Work out the finished part from the listing and answer in its coordinate system (mm). A direction names the side the tool comes from. Give positions to 0.01 mm unless a question says otherwise; leave off trailing zeros. Write each loop counter-clockwise with the first axis right and the second up, starting at its lowest first coordinate (ties: lowest second). Pieces come first, ordered by that corner, then holes. Notation, with made-up numbers: (19.5, -11.5) - (33.5, -11.5) arc R16 cw to (33.5, -3.5) - close; hole circle Ø8 at (41.25, 84). An arc over 180 degrees is marked (long way). Write each question's results on one line, items separated by ' | '. Start each with the question number.
from build123d import *

# Parameters (mm, degrees)
SKETCH4_W           = 260.35
SKETCH4_H           = 158.75
SKETCH4_W_2         = 254
SKETCH4_H_2         = 152.4
BOSS_EXTRUDE1_DEPTH = 38.1
SKETCH5_R           = 1.5875
CUT_EXTRUDE1_DEPTH  = 305.618044648
SKETCH5_4_R         = 1.5875
CUT_EXTRUDE2_DEPTH  = 305.618044648


with BuildPart() as part:
    # Sketch4 → Boss-Extrude1 (new body)
    with BuildSketch(Plane(origin=(0, 0, 0), x_dir=(1, 0, 0), z_dir=(0, 1, 0))):
        with Locations((127, 76.2)):
            Rectangle(SKETCH4_W, SKETCH4_H)
        with Locations((127, 76.2)):
            Rectangle(SKETCH4_W_2, SKETCH4_H_2, mode=Mode.SUBTRACT)
    extrude(amount=BOSS_EXTRUDE1_DEPTH)

    # Sketch5 → Cut-Extrude1 (cut, through all)
    with BuildSketch(Plane.XY.offset(3.175)):
        with Locations((92.075, 19.05)):
            Circle(SKETCH5_R)
    extrude(amount=-CUT_EXTRUDE1_DEPTH, mode=Mode.SUBTRACT)

    # Sketch5<4> → Cut-Extrude2 (cut, through all)
    with BuildSketch(Plane.XY.offset(3.175)):
        with Locations((161.925, 19.05)):
            Circle(SKETCH5_4_R)
    extrude(amount=-CUT_EXTRUDE2_DEPTH, mode=Mode.SUBTRACT)


solid = part.part
Q1. Given pin 1 (2.5 mm diameter, centred on x = 92.075, y = 19.05, fed in from +Z), flat-ended and moving along its own axis, determine where the tip first touches the part or whether it passes through.
Q2. The mould has two halves that part along Z. Classify faces 3 (the flat face through (0, 19, -75)), 4 (the flat face through (125, 19, 3.175)), 5 (the flat face through (-3.175, 19, -75)): pulls with the +Z half, pulls with the -Z half, needs draft (parallel to the pull), parting line crosses it, or undercut.
Q3. A cutting plane is placed at C-C, the plane y = 9.5. Write down the section's boundary in (x, z) (3 decimals).
Q4. A cutting plane is placed at B-B, the plane x = 169. Write down the section's boundary in (y, z) (3 decimals).
Q5. Consider L1, parallel to X at y = 19, z = -153 (3 decimals); L2, parallel to Z at x = 162.5, y = 2 (3 decimals); L3, parallel to X at y = 30, z = -104.5 (3 decimals). Determine where each line is inside the solid, lowest interval first.
Q6. A tool of negligible diameter and unlimited length cuts with its end or side. For faces 1 (the flat face through (257.175, 19, -75)), 2 (the flat face through (125, 19, 0)), from which of +Z, -Z, +X, -X, +Y, -Y can it reach the whole face along a straight path? Write none if from no direction.
Q7. A cutting plane is placed at A-A, the plane z = -50.5. Write down the section's boundary in (x, y) (3 decimals), and give its area (3 significant figures).
Result:
1) pin 1: passes through
2) face 3: undercut | face 4: pulls with the +Z half | face 5: needs draft
3) outline: (-3.175, -155.575) - (257.175, -155.575) - (257.175, 3.175) - (-3.175, 3.175) - close; hole (0, -152.4) - (254, -152.4) - (254, 0) - (0, 0) - close
4) outline: (0, -155.575) - (38.1, -155.575) - (38.1, -152.4) - (0, -152.4) - close; (0, 0) - (38.1, 0) - (38.1, 3.175) - (0, 3.175) - close
5) L1: x = -3.175 to 90.488, 93.662 to 160.338, 163.512 to 257.175 | L2: z = -155.575 to -152.4, 0 to 3.175 | L3: x = -3.175 to 0, 254 to 257.175
6) face 1: +Z, -Z, +X, +Y, -Y | face 2: +Y, -Y
7) outline: (-3.175, 0) - (0, 0) - (0, 38.1) - (-3.175, 38.1) - close; (254, 0) - (257.175, 0) - (257.175, 38.1) - (254, 38.1) - close | area: 242 mm2
